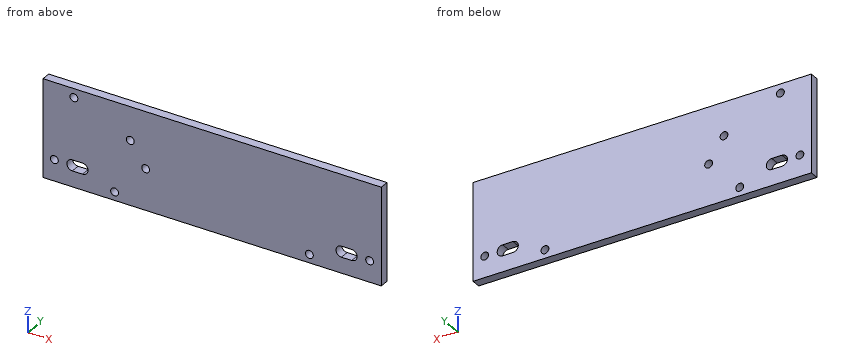
```python
from build123d import *

# Parameters (mm, degrees)
F0_W     = 419.1
F0_H     = 120.65
F1_DEPTH = 5.6261
F2_R     = 4.8387
F3_DEPTH = 11.2532
F5_DEPTH = 11.2532


with BuildPart() as f1:
    # F0 (on Front) → F1 (new body, symmetric)
    with BuildSketch(Plane.XZ):
        with Locations((209.55, 60.325)):
            Rectangle(F0_W, F0_H)
    extrude(amount=F1_DEPTH, both=True)

    # F2 (on face) → F3 (cut, through all)
    with BuildSketch(Plane.XZ.offset(5.6261)):
        with Locations((14.097, 26.2636)):
            Circle(F2_R)
        with Locations((38.3032, 109.601)):
            Circle(F2_R)
        with Locations((108.1532, 79.4512)):
            Circle(F2_R)
        with Locations((329.9968, 10.3886)):
            Circle(F2_R)
        with Locations((88.6968, 10.3886)):
            Circle(F2_R)
        with Locations((127.2032, 50.8762)):
            Circle(F2_R)
        with Locations((404.622, 26.2636)):
            Circle(F2_R)
    extrude(amount=-F3_DEPTH, mode=Mode.SUBTRACT)

    # F4 (on face) → F5 (cut, through all)
    with BuildSketch(Plane.XZ.offset(5.6261)):
        with BuildLine():
            Line((49.022, 33.0073), (36.322, 33.0073))
            ThreePointArc((36.322, 33.0073), (29.5783, 26.2636), (36.322, 19.5199))
            Line((36.322, 19.5199), (49.022, 19.5199))
            ThreePointArc((49.022, 19.5199), (55.7657, 26.2636), (49.022, 33.0073))
        make_face()
        with BuildLine():
            Line((382.397, 33.0073), (369.697, 33.0073))
            ThreePointArc((369.697, 33.0073), (362.9533, 26.2636), (369.697, 19.5199))
            Line((369.697, 19.5199), (382.397, 19.5199))
            ThreePointArc((382.397, 19.5199), (389.1407, 26.2636), (382.397, 33.0073))
        make_face()
    extrude(amount=-F5_DEPTH, mode=Mode.SUBTRACT)


solid = f1.part
```
Design review of the part built by this model. Coordinates are the model's own, in mm. Coordinates: 2 decimals unless noted, no trailing zeros. Answer as a JSON object with one key per item and string values.
Item 1: Add section A-A, the plane y = 2. State how many separate pieces and enclosed holes the cut face has, and give its area (3 significant figures).
Outcome:
{"separate pieces": "1", "enclosed holes": "9", "area": "49,400 mm²"}
Item 2: Insertion check: pin 1 Ø7.5 at (x, z) = (14.1, 26.26) entering from -Y. The pin has a flat end and moves straight along its axis. Give the tip position at first contact, or say it passes through.
Outcome:
{"pin 1": "through"}
Item 3: Wall thickness on probe 1 along Z at (x, y) = (127, 2.75); probe 2 along X at (y, z) = (-1, 27); probe 3 along Z at (x, y) = (371, -0.5): over which ranges is each line inside the solid? List them lowest first.
Outcome:
{"probe 1": "0 to 46.04, 55.71 to 120.65", "probe 2": "0 to 9.31, 18.88 to 29.62, 55.73 to 362.99, 389.1 to 399.84, 409.4 to 419.1", "probe 3": "0 to 19.52, 33.01 to 120.65"}
